Build history of the part. All positions in model axes, mm. Coordinates: 2 decimals unless noted, no trailing zeros. Write each loop counter-clockwise with the first axis right and the second up, starting at its lowest first coordinate (ties: lowest second). Pieces come first, ordered by that corner, then holes.
```python
from build123d import *

# Parameters (mm, degrees)
PAD_DEPTH    = 0.25
SKETCH001_R  = 0.75
PAD001_DEPTH = 0.25
SKETCH002_R  = 0.75
PAD002_DEPTH = 0.25
SKETCH003_R  = 0.75
PAD003_DEPTH = 0.25
SKETCH004_R  = 0.75
PAD004_DEPTH = 0.4
SKETCH005_W  = 10
SKETCH005_H  = 10
POCKET_DEPTH = 12.626


with BuildPart() as part:
    # Sketch (on DatumPlane) → Pad (new body, symmetric)
    with BuildSketch(Plane.XY.offset(0.5675)):
        Polygon((-7.195606, 5), (-7.195606, 0), (-7.195606, -5), (-6.795606, -5), (-6.395606, -5), (-6.395606, -0.4), (10, -0.4), (10, 0.4), (-6.395606, 0.4), (-6.395606, 5), (-6.795606, 5), align=None)
    extrude(amount=PAD_DEPTH, both=True)

    # Sketch001 (on DatumPlane) → Pad001 (join, symmetric)
    with BuildSketch(Plane.XY.offset(0.5675)):
        Circle(SKETCH001_R)
    extrude(amount=PAD001_DEPTH, both=True)

    # Sketch002 (on DatumPlane) → Pad002 (join, symmetric)
    with BuildSketch(Plane.XY.offset(0.5675)):
        with Locations((-6.795606, 5)):
            Circle(SKETCH002_R)
    extrude(amount=PAD002_DEPTH, both=True)

    # Sketch003 (on DatumPlane) → Pad003 (join, symmetric)
    with BuildSketch(Plane.XY.offset(0.5675)):
        with Locations((-6.795606, -5)):
            Circle(SKETCH003_R)
    extrude(amount=PAD003_DEPTH, both=True)

    # Sphere → Sphere (revolve, cut)
    with BuildSketch(Plane.XZ):
        with BuildLine():
            ThreePointArc((0, -0.635), (0.635, 0), (0, 0.635))
            Line((0, 0.635), (0, -0.635))
        make_face()
    revolve(axis=Axis((0, 0, 0), (0, 0, 1)), mode=Mode.SUBTRACT)

    # Sphere001 → Sphere001 (revolve, cut)
    with BuildSketch(Plane(origin=(-6.795606, 5, 1.135), x_dir=(1, 0, 0), z_dir=(0, -1, 0))):
        with BuildLine():
            ThreePointArc((0, -0.635), (0.635, 0), (0, 0.635))
            Line((0, 0.635), (0, -0.635))
        make_face()
    revolve(axis=Axis((-6.795606, 5, 1.135), (0, 0, 1)), mode=Mode.SUBTRACT)

    # Sphere002 → Sphere002 (revolve, cut)
    with BuildSketch(Plane(origin=(-6.795606, -5, 1.135), x_dir=(1, 0, 0), z_dir=(0, -1, 0))):
        with BuildLine():
            ThreePointArc((0, -0.635), (0.635, 0), (0, 0.635))
            Line((0, 0.635), (0, -0.635))
        make_face()
    revolve(axis=Axis((-6.795606, -5, 1.135), (0, 0, 1)), mode=Mode.SUBTRACT)

    # Sketch004 (on DatumPlane) → Pad004 (join, symmetric)
    with BuildSketch(Plane(origin=(0, 0, 0.5675), x_dir=(1, 0, 0), z_dir=(0, -1, 0))):
        with Locations((6.8, 0)):
            Circle(SKETCH004_R)
    extrude(amount=PAD004_DEPTH, both=True)

    # Sphere003 → Sphere003 (revolve, cut)
    with BuildSketch(Plane(origin=(6.8, 0.7175, 0.5675), x_dir=(1, 0, 0), z_dir=(0, -1, 0))):
        with BuildLine():
            ThreePointArc((0, -0.635), (0.635, 0), (0, 0.635))
            Line((0, 0.635), (0, -0.635))
        make_face()
    revolve(axis=Axis((6.8, 0.7175, 0.5675), (0, 0, 1)), mode=Mode.SUBTRACT)

    # Sketch005 (on DatumPlane) → Pocket (cut, through all)
    with BuildSketch(Plane(origin=(-2.625, 0, 0), x_dir=(0, -1, 0), z_dir=(-1, 0, 0))):
        Rectangle(SKETCH005_W, SKETCH005_H)
    extrude(amount=-POCKET_DEPTH, mode=Mode.SUBTRACT)


solid = part.part
```
1. Mould opens along Y. For faces 1 (the face through (-6, 0, 0.318)), 2 (the face through (-6.77, 5.75, 0.57)) say: +Y half, -Y half, draft (parallel to the pull), parting line (faces both ways), or undercut.
Computed values:
face 1: draft
face 2: undercut
2. Saw through at C-C on x = -5.45. List the corners of the cut face in (y, z), plus the area to 3 significant figures.
Computed values:
outline: (-0.4, 0.32) - (0.4, 0.32) - (0.4, 0.82) - (-0.4, 0.82) - close
area: 0.400 mm2
3. Saw through at A-A on z = 0.65. List the corners of the cut face in (x, y) (3 decimals), plus the area to 3 significant figures.
Computed values:
outline: (-7.196, -4.366) arc R0.75 ccw (long way) to (-6.396, -4.366) - (-6.396, -0.4) - (-2.625, -0.4) - (-2.625, 0.4) - (-6.396, 0.4) - (-6.396, 4.366) arc R0.75 ccw (long way) to (-7.196, 4.366) - close; hole circle Ø0.82 at (-6.796, -5); hole circle Ø0.82 at (-6.796, 5)
area: 12.4 mm2
4. Probe line 1 along Y through (x, z) = (-5.25, 0.75); line 2 along X through (y, z) = (3, 0.45); line 3 along X through (y, z) = (-5, 0.7). List the from-to ranges inside material, lowest first.
Computed values:
line 1: y = -0.4 to 0.4
line 2: x = -7.2 to -6.4
line 3: x = -7.55 to -7.26, -6.33 to -6.05
5. Flat gauge pins, fed straight in: pin 1 (1.5 mm diameter, centred on x = -4.5, y = -1.5, fed in from +Z); pin 2 (1 mm diameter, centred on x = -6, y = -0.5, fed in from +Z). Where does each tip first touch, or does it go through?
Computed values:
pin 1: passes through
pin 2: stops at z = 0.82
